Source: three-view drawing plus pictorial views. Frame: mm from the lowest corner of the part. A direction names the side the tool comes from. Coordinates: 2 decimals unless noted, no trailing zeros. Write each loop counter-clockwise with the first axis right and the second up, starting at its lowest first coordinate (ties: lowest second). Pieces come first, ordered by that corner, then holes. Notation, with made-up numbers: (68.5, 17) - (74.5, 17) arc R22 cw to (74.5, 30) - close; hole circle Ø5 at (89.25, 12). An arc over 180 degrees is marked (long way). Put each result on its own line as item: value.
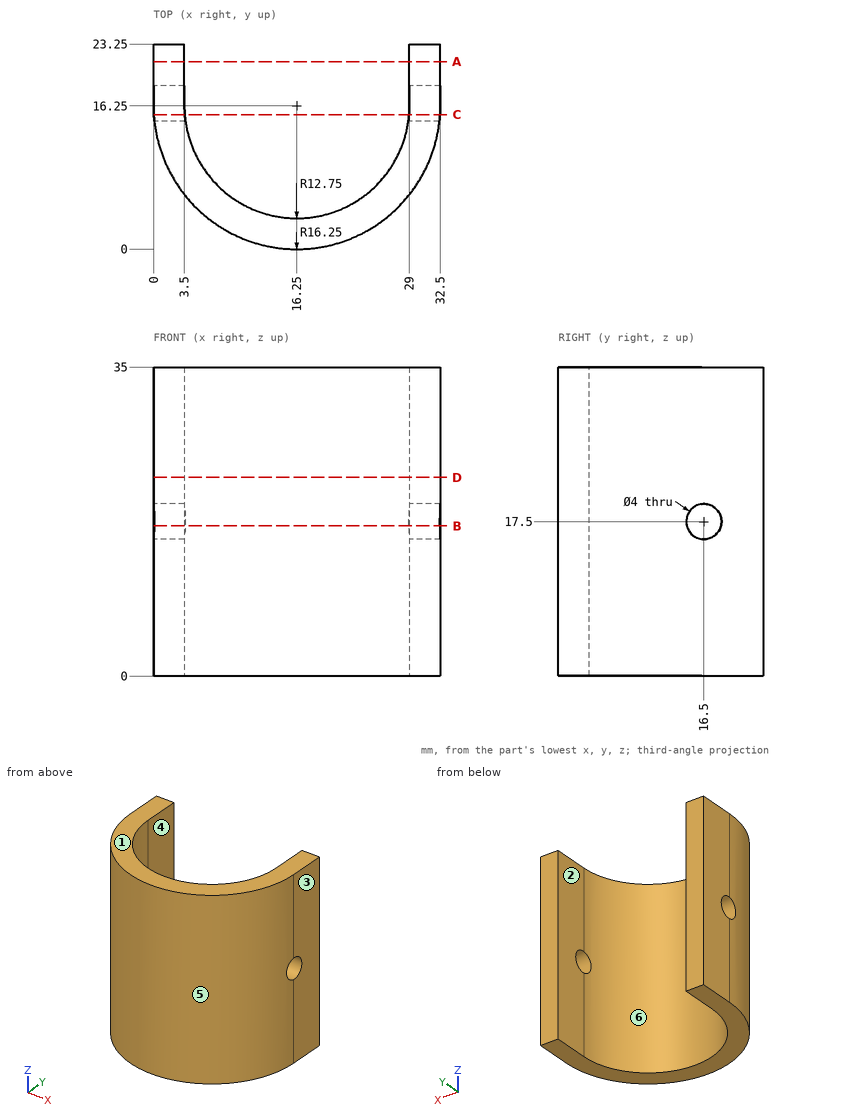
1. Section query A-A (y = 21.25). Return loops of the section in (x, z).
Answer below:
outline: (0, 0) - (3.5, 0) - (3.5, 35) - (0, 35) - close; (29, 0) - (32.5, 0) - (32.5, 35) - (29, 35) - close
2. Mould query, pull axis X, two halves, no side actions, for the marked faces 3, 4, 5 and 6. Classes: +X half, -X half, draft (parallel to the pull), parting line (faces both ways), or undercut.
Answer below:
face 3: +X half
face 4: undercut
face 5: parting line
face 6: undercut
3. Set-up query: the marked faces 1 and 2. Return all of +Z, -Z, +X, -X, +Y, -Y with unobstructed straight access to the full face (end or side cutting, diameter ignored); none if empty.
Answer below:
face 1: +Z, +X, -X, +Y, -Y
face 2: +Z, -Z, +Y
4. Pin query (flat end, axial travel): pin 1 Ø5 at (y, z) = (10.5, 28) entering from +X; pin 2 Ø8 at (x, z) = (10.5, 29) entering from +Y; pin 3 Ø5 at (y, z) = (7.5, 10) entering from +X; pin 4 Ø10 at (x, y) = (21, 19) entering from -Z. Return the tip coordinate at first contact, or that it passes through.
Answer below:
pin 1: stops at x = 32.17
pin 2: stops at y = 8.03
pin 3: stops at x = 31.25
pin 4: passes through
5. Section query B-B (z = 17). Return loops of the section in (x, y).
Answer below:
outline: (0, 18.44) - (3.5, 18.44) - (3.5, 23.25) - (0, 23.25) - close; (0.09, 14.56) arc R16.25 ccw to (32.41, 14.56) - (28.89, 14.56) arc R12.75 cw to (3.61, 14.56) - close; (29, 18.44) - (32.5, 18.44) - (32.5, 23.25) - (29, 23.25) - close
6. Ray query, probe 1 along Z at (x, y) = (31.6, 16.5); probe 2 along X at (y, z) = (12.5, 8.5); probe 3 along X at (y, z) = (21, 30). Return the intervals inside material, ascending. Write a range as from..to.
Answer below:
probe 1: z = 0..15.5, 19.5..35
probe 2: x = 0.44..4.06, 28.44..32.06
probe 3: x = 0..3.5, 29..32.5
7. Section query C-C (y = 15.25). Return loops of the section in (x, z), then the cut area to 3 significant figures.
Answer below:
outline: (0.03, 0) - (3.54, 0) - (3.54, 15.94) - (0.03, 15.94) - close; (0.03, 19.06) - (3.54, 19.06) - (3.54, 35) - (0.03, 35) - close; (28.96, 0) - (32.47, 0) - (32.47, 15.94) - (28.96, 15.94) - close; (28.96, 19.06) - (32.47, 19.06) - (32.47, 35) - (28.96, 35) - close
area: 224 mm²
8. Section query D-D (z = 22.5). Return loops of the section in (x, y), then the cut area to 3 significant figures.
Answer below:
outline: (0, 16.25) arc R16.25 ccw to (32.5, 16.25) - (32.5, 23.25) - (29, 23.25) - (29, 16.25) arc R12.75 cw to (3.5, 16.25) - (3.5, 23.25) - (0, 23.25) - close
area: 208 mm²
